Model file for the job. Use its own axes, mm. Face numbers are marked on the shaded views. A direction names the side the tool comes from. Coordinates: 2 decimals unless noted, no trailing zeros. Order: outer loops, then holes, each group sorted by start corner. A loop starts at its lowest first (then second) coordinate and runs counter-clockwise, first axis right, second up. Notation, with made-up numbers: (-31.5, -12) -> (-19.5, -12) arc R24 cw to (-19.5, 8) -> close; hole circle Ø11 at (1, 39). An arc over 180 degrees is marked (long way). Write item = value, one per line. Start each with the question number.
Q1. Mould opens along Y. For the marked faces 5, 6, 7 and 8 say: +Y half, -Y half, draft (parallel to the pull), parting line (faces both ways), or undercut.
Q2. Cut at D-D, the plane x = 21. List the corners of the cut face in (y, z), plus the area to 3 significant figures.
Q3. Cut at B-B, the plane z = -28. List the corners of the cut face in (x, y).
Q4. 3-axis set-ups, long thin cutter, end or side, ignore diameter. For the marked faces 1, 2, 3 and 4: which of +Z, -Z, +X, -X, +Y, -Y reach the whole face in a straight line?
Q5. Cut at A-A, the plane x = -23.5. List the corners of the cut face in (y, z).
Q6. Wall check: line 1 (Z direction, x = -20, y = 9); line 2 (X direction, y = 6.5, z = 40); line 3 (X direction, y = 13.75, z = -7). Give the ranges that are in metal, low to high. Write a range as from..to.
Q7. Cut at C-C, the plane x = 44. List the corners of the cut face in (y, z).
Q8. Flat gauge pins, fed straight in: pin 1 (4 mm diameter, centred on x = 30.5, y = 5, fed in from -Z); pin 2 (4 mm diameter, centred on x = -39.5, y = 10, fed in from -Z); pin 3 (8 mm diameter, centred on x = 27, z = 16.5, fed in from +Y). Where does each tip first touch, or does it go through?
from build123d import *

# Parameters (mm, degrees)
ESBO_O1_W                = 100
ESBO_O1_H                = 100
RESSALTO_EXTRUS_O1_DEPTH = 1.4
ESBO_O2_W                = 88
ESBO_O2_H                = 88
RESSALTO_EXTRUS_O2_DEPTH = 24
ESBO_O4_W                = 100
ESBO_O4_H                = 100
ESBO_O4_W_2              = 14.578639588
ESBO_O4_H_2              = 8.540496419
ESBO_O4_W_3              = 7.289319794
ESBO_O4_H_3              = 22.779124356
ESBO_O4_W_4              = 18.794478339
ESBO_O4_H_4              = 37.364152615
ESBO_O4_W_5              = 26.546651383
ESBO_O4_H_5              = 38.188932231
ESBO_O4_W_6              = 20.632673902
ESBO_O4_H_6              = 13.495583341
ESBO_O4_W_7              = 9.670550534
ESBO_O4_H_7              = 6
ESBO_O4_W_8              = 9.833990962
ESBO_O4_H_8              = 4.968111267
CORTE_EXTRUS_O1_DEPTH    = 24
ESBO_O5_W                = 26.546651383
ESBO_O5_H                = 38.188932231
ESBO_O5_W_2              = 7.289319794
ESBO_O5_H_2              = 22.779124356
ESBO_O5_W_3              = 20.632673902
ESBO_O5_H_3              = 13.495583341
ESBO_O5_W_4              = 14.578639588
ESBO_O5_H_4              = 8.540496419
ESBO_O5_W_5              = 9.670550534
ESBO_O5_H_5              = 6
ESBO_O5_W_6              = 9.833990962
ESBO_O5_H_6              = 4.968111267
CORTE_EXTRUS_O2_DEPTH    = 10
ESBO_O6_R                = 2
CORTE_EXTRUS_O3_DEPTH    = 1
CHANFRO1_SIZE            = 1.5
CORTE_EXTRUS_O4_REACH    = 102.636
ESBO_O7_W                = 33.364152615
ESBO_O7_H                = 10
CORTE_EXTRUS_O5_REACH    = 111.458
ESBO_O8_W                = 22.546651383
ESBO_O8_H                = 10.000703343
CORTE_EXTRUS_O6_REACH    = 101.657
ESBO_O9_W                = 9.495583341
ESBO_O9_H                = 10
ESBO_O10_W               = 3
ESBO_O10_H               = 10
CORTE_EXTRUS_O7_DEPTH    = 9.670550534
CORTE_EXTRUS_O8_REACH    = 97.616
ESBO_O11_W               = 2.484055633
ESBO_O11_H               = 10
ESBO_O12_R               = 1.75
CORTE_EXTRUS_O9_DEPTH    = 1.4
RESSALTO_EXTRUS_O3_DEPTH = 11


with BuildPart() as part:
    # Esboço1 → Ressalto-extrusão1 (new body)
    with BuildSketch(Plane(origin=(0, 0, 0), x_dir=(1, 0, 0), z_dir=(0, 1, 0))):
        Rectangle(ESBO_O1_W, ESBO_O1_H)
    extrude(amount=RESSALTO_EXTRUS_O1_DEPTH)

    # Esboço2 → Ressalto-extrusão2 (add)
    with BuildSketch(Plane(origin=(0, 1.4, 0), x_dir=(1, 0, 0), z_dir=(0, 1, 0))):
        Rectangle(ESBO_O2_W, ESBO_O2_H)
    extrude(amount=RESSALTO_EXTRUS_O2_DEPTH)

    # Esboço4 → Corte-extrusão1 (cut)
    with BuildSketch(Plane(origin=(0, 25.4, 0), x_dir=(1, 0, 0), z_dir=(0, 1, 0))):
        Rectangle(ESBO_O4_W, ESBO_O4_H)
        with Locations((31.283330783, -39.729751791)):
            Rectangle(ESBO_O4_W_2, ESBO_O4_H_2, mode=Mode.SUBTRACT)
        with Locations((27.638670886, -17.539925754)):
            Rectangle(ESBO_O4_W_3, ESBO_O4_H_3, mode=Mode.SUBTRACT)
        with Locations((24.164004049, 23.617553252)):
            Rectangle(ESBO_O4_W_4, ESBO_O4_H_4, mode=Mode.SUBTRACT)
        with Locations((-16.396734338, 24.905533884)):
            Rectangle(ESBO_O4_W_5, ESBO_O4_H_5, mode=Mode.SUBTRACT)
        with Locations((-22.063064097, -29.56405701)):
            Rectangle(ESBO_O4_W_6, ESBO_O4_H_6, mode=Mode.SUBTRACT)
        with Locations((7.531276247, -29.56405701)):
            Rectangle(ESBO_O4_W_6, ESBO_O4_H_6, mode=Mode.SUBTRACT)
        with Locations((-39.164724733, 33)):
            Rectangle(ESBO_O4_W_7, ESBO_O4_H_7, mode=Mode.SUBTRACT)
        with Locations((-39.164724733, 16)):
            Rectangle(ESBO_O4_W_7, ESBO_O4_H_7, mode=Mode.SUBTRACT)
        with Locations((-39.164724733, -1)):
            Rectangle(ESBO_O4_W_7, ESBO_O4_H_7, mode=Mode.SUBTRACT)
        with Locations((-39.164724733, -18)):
            Rectangle(ESBO_O4_W_7, ESBO_O4_H_7, mode=Mode.SUBTRACT)
        with Locations((-22.524725577, -41.515944367)):
            Rectangle(ESBO_O4_W_8, ESBO_O4_H_8, mode=Mode.SUBTRACT)
        with Locations((7.992937727, -41.515944367)):
            Rectangle(ESBO_O4_W_8, ESBO_O4_H_8, mode=Mode.SUBTRACT)
    extrude(amount=-CORTE_EXTRUS_O1_DEPTH, mode=Mode.SUBTRACT)

    # Esboço5 → Corte-extrusão2 (cut)
    with BuildSketch(Plane(origin=(0, 25.4, 0), x_dir=(1, 0, 0), z_dir=(0, 1, 0))):
        with Locations((-16.396734338, 24.905533884)):
            Rectangle(ESBO_O5_W, ESBO_O5_H)
        with Locations((27.638670886, -17.539925754)):
            Rectangle(ESBO_O5_W_2, ESBO_O5_H_2)
        with Locations((7.531276247, -29.56405701)):
            Rectangle(ESBO_O5_W_3, ESBO_O5_H_3)
        with Locations((-22.063064097, -29.56405701)):
            Rectangle(ESBO_O5_W_3, ESBO_O5_H_3)
        with Locations((31.283330783, -39.729751791)):
            Rectangle(ESBO_O5_W_4, ESBO_O5_H_4)
        with Locations((-39.164724733, -18)):
            Rectangle(ESBO_O5_W_5, ESBO_O5_H_5)
        with Locations((-39.164724733, -1)):
            Rectangle(ESBO_O5_W_5, ESBO_O5_H_5)
        with Locations((-39.164724733, 16)):
            Rectangle(ESBO_O5_W_5, ESBO_O5_H_5)
        with Locations((-39.164724733, 33)):
            Rectangle(ESBO_O5_W_5, ESBO_O5_H_5)
        with Locations((7.992937727, -41.515944367)):
            Rectangle(ESBO_O5_W_6, ESBO_O5_H_6)
        with Locations((-22.524725577, -41.515944367)):
            Rectangle(ESBO_O5_W_6, ESBO_O5_H_6)
    extrude(amount=-CORTE_EXTRUS_O2_DEPTH, mode=Mode.SUBTRACT)

    # Esboço6 → Corte-extrusão3 (cut)
    with BuildSketch(Plane(origin=(0, 15.4, 0), x_dir=(1, 0, 0), z_dir=(0, 1, 0))):
        with Locations(Location((27.283330783, -39.729751791, 0), (0, 0, 270))):
            Circle(ESBO_O6_R)
        with Locations(Location((35.283330783, -39.729751791, 0), (0, 0, 270))):
            Circle(ESBO_O6_R)
    extrude(amount=-CORTE_EXTRUS_O3_DEPTH, mode=Mode.SUBTRACT)

    # Chanfro1
    chanfro1_edges = [part.edges().sort_by_distance(p)[0] for p in [
        (31.283330783, 15.4, 35.459503581),
    ]]
    chamfer(chanfro1_edges, length=CHANFRO1_SIZE)

    # Esboço7 → Corte-extrusão4 (cut, up to next)
    with BuildSketch(Plane(origin=(33.561243218, 0, 0), x_dir=(0, 0, -1), z_dir=(1, 0, 0)), mode=Mode.PRIVATE) as corte_extrus_o4_sk1:
        with Locations((23.617553252, 6.4)):
            Rectangle(ESBO_O7_W, ESBO_O7_H)
    corte_extrus_o4_tool1 = extrude(corte_extrus_o4_sk1.sketch, amount=-CORTE_EXTRUS_O4_REACH, mode=Mode.PRIVATE) & part.part
    add(corte_extrus_o4_tool1.solids().sort_by_distance((33.561243, 6.4, -23.617553))[0], mode=Mode.SUBTRACT)

    # Esboço8 → Corte-extrusão5 (cut, up to next)
    with BuildSketch(Plane(origin=(0, 0, -44), x_dir=(-1, 0, 0), z_dir=(0, 0, -1)), mode=Mode.PRIVATE) as corte_extrus_o5_sk1:
        with Locations((16.396734338, 6.400351672)):
            Rectangle(ESBO_O8_W, ESBO_O8_H)
    corte_extrus_o5_tool1 = extrude(corte_extrus_o5_sk1.sketch, amount=-CORTE_EXTRUS_O5_REACH, mode=Mode.PRIVATE) & part.part
    add(corte_extrus_o5_tool1.solids().sort_by_distance((-16.396734, 6.400352, -44))[0], mode=Mode.SUBTRACT)

    # Corte-extrusão6: up to this face of the body (flat: up to its plane)
    corte_extrus_o6_end = Plane(part.part.faces().sort_by_distance((17.847613198, 8.4, 29.56405701))[0])
    # Esboço9 → Corte-extrusão6 (cut, up to the picked face)
    with BuildSketch(Plane.ZY.offset(32.379401048), mode=Mode.PRIVATE) as corte_extrus_o6_sk1:
        with Locations((29.56405701, 6.4)):
            Rectangle(ESBO_O9_W, ESBO_O9_H)
    corte_extrus_o6_tool1 = split(extrude(corte_extrus_o6_sk1.sketch, amount=-CORTE_EXTRUS_O6_REACH, mode=Mode.PRIVATE), bisect_by=corte_extrus_o6_end, keep=Keep.BOTH, mode=Mode.PRIVATE)
    add(corte_extrus_o6_tool1.solids().sort_by(Axis((-32.379401, 6.4, 29.564057), (1, 0, 0)))[0], mode=Mode.SUBTRACT)

    # Esboço10 → Corte-extrusão7 (cut)
    with BuildSketch(Plane.ZY.offset(34.329449466)):
        with Locations((-31.5, 10.4)):
            Rectangle(ESBO_O10_W, ESBO_O10_H)
        with Locations((-14.5, 10.4)):
            Rectangle(ESBO_O10_W, ESBO_O10_H)
        with Locations((2.5, 10.4)):
            Rectangle(ESBO_O10_W, ESBO_O10_H)
        with Locations((19.5, 10.4)):
            Rectangle(ESBO_O10_W, ESBO_O10_H)
    extrude(amount=CORTE_EXTRUS_O7_DEPTH, mode=Mode.SUBTRACT)

    # Corte-extrusão8: up to this face of the body (flat: up to its plane)
    corte_extrus_o8_end = Plane(part.part.faces().sort_by_distance((12.909933208, 8.4, 41.515944367))[0])
    # Esboço11 → Corte-extrusão8 (cut, up to the picked face)
    with BuildSketch(Plane.ZY.offset(27.441721058), mode=Mode.PRIVATE) as corte_extrus_o8_sk1:
        with Locations((42.757972184, 10.4)):
            Rectangle(ESBO_O11_W, ESBO_O11_H)
    corte_extrus_o8_tool1 = split(extrude(corte_extrus_o8_sk1.sketch, amount=-CORTE_EXTRUS_O8_REACH, mode=Mode.PRIVATE), bisect_by=corte_extrus_o8_end, keep=Keep.BOTH, mode=Mode.PRIVATE)
    add(corte_extrus_o8_tool1.solids().sort_by(Axis((-27.441721, 10.4, 42.757972), (1, 0, 0)))[0], mode=Mode.SUBTRACT)

    # Esboço12 → Corte-extrusão9 (cut)
    with BuildSketch(Plane.XZ):
        with Locations(Location((-44, 40, 0), (0, 0, 270))):
            Circle(ESBO_O12_R)
        with Locations(Location((44, 40, 0), (0, 0, 270))):
            Circle(ESBO_O12_R)
        with Locations(Location((44, -40, 0), (0, 0, 270))):
            Circle(ESBO_O12_R)
        with Locations(Location((-44, -40, 0), (0, 0, 270))):
            Circle(ESBO_O12_R)
    extrude(amount=-CORTE_EXTRUS_O9_DEPTH, mode=Mode.SUBTRACT)

    # Esboço13 → Ressalto-extrusão3 (add)
    with BuildSketch(Plane(origin=(0, 0, -44), x_dir=(-1, 0, 0), z_dir=(0, 0, -1))):
        Polygon((5.123408647, 11.400703343), (27.67006003, 11.400703343), (27.67006003, 1.4), (29.67006003, 1.4), (29.67006003, 15.4), (3.123408647, 15.4), (3.123408647, 1.4), (5.123408647, 1.4), align=None)
    extrude(amount=RESSALTO_EXTRUS_O3_DEPTH)


solid = part.part
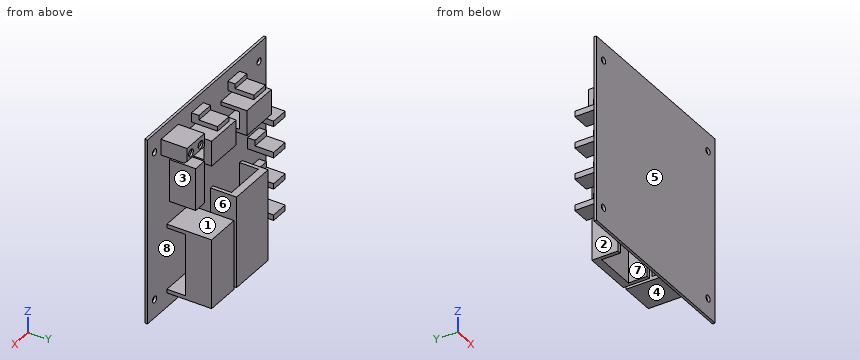
Here are the results:
q1.face_5 = -Y half
q1.face_6 = draft
q1.face_7 = undercut
q1.face_8 = undercut
q2.outline = (0, -50) -> (1.4, -50) -> (1.4, -42.3) -> (25.4, -42.3) -> (25.4, -4.94) -> (1.4, -4.94) -> (1.4, 50) -> (0, 50) -> close; hole (1.4, -40.3) -> (11.4, -40.3) -> (11.4, -6.94) -> (1.4, -6.94) -> close
q2.area = 703 mm²
q3.outline = (-50, 0) -> (50, 0) -> (50, 1.4) -> (-3.12, 1.4) -> (-3.12, 15.4) -> (-29.67, 15.4) -> (-29.67, 1.4) -> (-50, 1.4) -> close; (14.77, 11.4) -> (33.56, 11.4) -> (33.56, 25.4) -> (14.77, 25.4) -> close; hole (-27.67, 1.4) -> (-5.12, 1.4) -> (-5.12, 11.4) -> (-27.67, 11.4) -> close
q4.face_1 = +X, -X, +Y
q4.face_2 = -Z, +Y
q4.face_3 = +X, +Y
q4.face_4 = -Z, +X, +Y
q5.outline = (0, -50) -> (1.4, -50) -> (1.4, 22.82) -> (15.4, 22.82) -> (15.4, 36.31) -> (1.4, 36.31) -> (1.4, 39.03) -> (15.4, 39.03) -> (15.4, 41.52) -> (5.4, 41.52) -> (5.4, 44) -> (1.4, 44) -> (1.4, 50) -> (0, 50) -> close; (11.4, -55) -> (15.4, -55) -> (15.4, -5.81) -> (11.4, -5.81) -> close; hole (1.4, 24.82) -> (11.4, 24.82) -> (11.4, 34.31) -> (1.4, 34.31) -> close
q6.line_1 = 22.82..24.82, 34.31..36.31, 39.03..41.52
q6.line_2 = -27.44..-17.61, 3.08..12.91, 23.99..38.57
q6.line_3 = -29.67..-3.12, 14.77..33.56
q7.outline = (0, -50) -> (1.4, -50) -> (1.4, -41.75) -> (0, -41.75) -> close; (0, -38.25) -> (1.4, -38.25) -> (1.4, 38.25) -> (0, 38.25) -> close; (0, 41.75) -> (1.4, 41.75) -> (1.4, 50) -> (0, 50) -> close
q8.pin_1 = -42.3
q8.pin_2 = -36
q8.pin_3 = 15.4
